Verification items for the finished model (mm, model axes). A direction names the side the tool comes from. Round coordinates to 2 decimals unless told otherwise and drop trailing zeros. Loops run counter-clockwise (first coordinate to the right, second up) from the corner with the lowest first, then second, coordinate; pieces in that order, holes last. Notation, with made-up numbers: (31.5, 52.25) - (50.5, 52.25) arc R15 cw to (50.5, 79.25) - close; hole circle Ø11 at (-39.75, 43.5). An arc over 180 degrees is marked (long way). Use CSV: the item, a comma, the result in double quotes.
```python
from build123d import *

# Parameters (mm, degrees)
SKETCH1_R           = 4
BOSS_EXTRUDE1_DEPTH = 6
BOSS_EXTRUDE2_START = -6
SKETCH2_R           = 4
BOSS_EXTRUDE2_DEPTH = 6
FILLET1_R           = 5
SKETCH3_R           = 1.5
CUT_EXTRUDE1_DEPTH  = 19
SKETCH4_R           = 1.5
CUT_EXTRUDE2_DEPTH  = 19
FILLET2_R           = 100


with BuildPart() as part:
    # Sketch1 → Boss-Extrude1 (new body)
    with BuildSketch(Plane(origin=(0, 0, 0), x_dir=(1, 0, 0), z_dir=(0, 1, 0))):
        with BuildLine():
            Line((0, -17.5), (127.759093916, -17.5))
            ThreePointArc((127.759093916, -17.5), (163.75, 0), (127.759093916, 17.5))
            Line((127.759093916, 17.5), (0, 17.5))
            ThreePointArc((0, 17.5), (-17.5, 0), (0, -17.5))
        make_face()
        with Locations(Location((141.5, 0, 0), (0, 0, 270))):
            Circle(SKETCH1_R, mode=Mode.SUBTRACT)
        with Locations(Location((0, 0, 0), (0, 0, 270))):
            Circle(SKETCH1_R, mode=Mode.SUBTRACT)
    extrude(amount=BOSS_EXTRUDE1_DEPTH)

    # Sketch2 → Boss-Extrude2 (add)
    with BuildSketch(Plane(origin=(0, 6, 0), x_dir=(1, 0, 0), z_dir=(0, 1, 0)).offset(BOSS_EXTRUDE2_START)):
        with BuildLine():
            ThreePointArc((0, -22.5), (22.5, 0), (0, 22.5))
            Line((0, 22.5), (-76, 22.5))
            Line((-76, 22.5), (-76, -22.5))
            Line((-76, -22.5), (0, -22.5))
        make_face()
        with BuildLine():
            Line((-64.5, -17), (-69.5, -17))
            ThreePointArc((-69.5, -17), (-71, -15.5), (-69.5, -14))
            Line((-69.5, -14), (-64.5, -14))
            ThreePointArc((-64.5, -14), (-63, -15.5), (-64.5, -17))
        make_face(mode=Mode.SUBTRACT)
        with BuildLine():
            Line((-38.5, -14), (-37.5, -14))
            Line((-37.5, -14), (-33.5, -14))
            ThreePointArc((-33.5, -14), (-32, -15.5), (-33.5, -17))
            Line((-33.5, -17), (-38.5, -17))
            ThreePointArc((-38.5, -17), (-40, -15.5), (-38.5, -14))
        make_face(mode=Mode.SUBTRACT)
        with BuildLine():
            ThreePointArc((-49, 11), (-38.531049744, 3.376548613), (-42.572923734, -8.927076266))
            ThreePointArc((-42.572923734, -8.927076266), (-45.623451387, -10.468950256), (-49, -11))
            Line((-49, -11), (-54, -11))
            ThreePointArc((-54, -11), (-61.778174593, -7.778174593), (-65, 0))
            ThreePointArc((-65, 0), (-61.778174593, 7.778174593), (-54, 11))
            Line((-54, 11), (-49, 11))
        make_face(mode=Mode.SUBTRACT)
        with BuildLine():
            ThreePointArc((-64.5, 17), (-63, 15.5), (-64.5, 14))
            Line((-64.5, 14), (-69.5, 14))
            ThreePointArc((-69.5, 14), (-71, 15.5), (-69.5, 17))
            Line((-69.5, 17), (-64.5, 17))
        make_face(mode=Mode.SUBTRACT)
        with BuildLine():
            ThreePointArc((-33.5, 17), (-32, 15.5), (-33.5, 14))
            Line((-33.5, 14), (-38.5, 14))
            ThreePointArc((-38.5, 14), (-40, 15.5), (-38.5, 17))
            Line((-38.5, 17), (-33.5, 17))
        make_face(mode=Mode.SUBTRACT)
        with Locations(Location((0, 0, 0), (0, 0, 270))):
            Circle(SKETCH2_R, mode=Mode.SUBTRACT)
    extrude(amount=BOSS_EXTRUDE2_DEPTH)

    # Fillet1
    fillet1_edges = [part.edges().sort_by_distance(p)[0] for p in [
        (-76, 3, 22.5),
        (-76, 3, -22.5),
    ]]
    fillet(fillet1_edges, radius=FILLET1_R)

    # Sketch3 → Cut-Extrude1 (cut)
    with BuildSketch(Plane(origin=(0, 6, 0), x_dir=(1, 0, 0), z_dir=(0, 1, 0))):
        with Locations(Location((0, 12.5, 0), (0, 0, 270))):
            Circle(SKETCH3_R)
        with Locations(Location((12.5, 0, 0), (0, 0, 270))):
            Circle(SKETCH3_R)
        with Locations(Location((0, -12.5, 0), (0, 0, 270))):
            Circle(SKETCH3_R)
        with Locations(Location((-12.5, 0, 0), (0, 0, 270))):
            Circle(SKETCH3_R)
    extrude(amount=-CUT_EXTRUDE1_DEPTH, mode=Mode.SUBTRACT)

    # Sketch4 → Cut-Extrude2 (cut)
    with BuildSketch(Plane(origin=(0, 6, 0), x_dir=(1, 0, 0), z_dir=(0, 1, 0))):
        with Locations(Location((158.75, 0, 0), (0, 0, 270))):
            Circle(SKETCH4_R)
        with Locations(Location((141.5, -17.25, 0), (0, 0, 270))):
            Circle(SKETCH4_R)
        with Locations(Location((124.25, 0, 0), (0, 0, 270))):
            Circle(SKETCH4_R)
        with Locations(Location((141.5, 17.25, 0), (0, 0, 270))):
            Circle(SKETCH4_R)
    extrude(amount=-CUT_EXTRUDE2_DEPTH, mode=Mode.SUBTRACT)

    # Fillet2
    fillet2_edges = [part.edges().sort_by_distance(p)[0] for p in [
        (127.759093916, 3, -17.5),
        (127.759093916, 3, 17.5),
        (14.142135624, 3, -17.5),
        (14.142135624, 3, 17.5),
    ]]
    fillet(fillet2_edges, radius=FILLET2_R)


solid = part.part
```
1) Cross-section at A-A, the plane y = 3.2. Count the separate pieces of the cut face and the enclosed holes in it, then the cut area to 3 significant figures.
Returned:
separate pieces,"1"
enclosed holes,"15"
area,"8,670 mm²"
2) Mould release check, pull along Z, two halves, no side actions. Record for faces 6 (the face through (-67, 3, -14)), 7 (the face through (145.466, 2.958, -0.521)), 8 (the face through (3.17, 2.958, 22.276)), 9 (the face through (20.554, 2.958, -18.497)): +Z half, -Z half, draft (parallel to the pull), parting line (faces both ways), or undercut.
Returned:
face 6,"undercut"
face 7,"undercut"
face 8,"+Z half"
face 9,"-Z half"
3) Cross-section at B-B, the plane x = 70.5. Record the cut outline in (y, z).
Returned:
outline,"(0, -17.5) - (6, -17.5) - (6, 17.5) - (0, 17.5) - close"
4) Access from +Z, -Z, +X, -X, +Y, -Y to the whole of each face (thin tool, end or side, straight path). Record for faces 1 (the face through (121.886, 3.042, -18.504)), 2 (the face through (-36, 3, 22.5)), 3 (the face through (-36, 3, 17)), 4 (the face through (121.5, 3.04, 18.45)), 5 (the face through (-74.5, 3.04, 21.07)).
Returned:
face 1,"-Z, +Y, -Y"
face 2,"+Z, +X, -X, +Y, -Y"
face 3,"+Y, -Y"
face 4,"+Z, +Y, -Y"
face 5,"+Z, -X, +Y, -Y"
5) Cross-section at C-C, the plane x = 26.5. Record the cut outline in (y, z), then the cut area to 3 significant figures.
Returned:
outline,"(0, -17.83) - (6, -17.83) - (6, 17.83) - (0, 17.83) - close"
area,"214 mm²"
6) Gauge pin test, flat ends, axial feed: pin 1 Ø3 at (y, z) = (1, -17.5) entering from +X; pin 2 Ø2 at (x, y) = (68, 2) entering from -Z; pin 3 Ø2 at (y, z) = (2, -15.5) entering from +X. Record the tip position at first contact, or that the pin passes through.
Returned:
pin 1,"stops at x = 156.96"
pin 2,"stops at z = -17.5"
pin 3,"stops at x = 158.38"
7) Thickness scan on probe 1 along Z at (x, y) = (-49, 5.4); probe 2 along X at (y, z) = (3.85, 16); probe 3 along X at (y, z) = (0.35, -3). Record the ranges inside material, lowest first. Write a range as [from, to].
Returned:
probe 1,"z = [-22.5, -11], [11, 22.5]"
probe 2,"x = [-76, -70.91], [-63.09, -39.91], [-32.09, 140.67], [142.33, 156.96]"
probe 3,"x = [-76, -64.58], [-38.42, -2.65], [2.65, 138.85], [144.15, 163.55]"
